```python
from build123d import *

# Parameters (mm, degrees)
SKETCH_1_R               = 25
SKETCH_1_R_2             = 12
EXTRUDE_1_DEPTH          = 10
SKETCH_2_R               = 25
SKETCH_2_R_2             = 4
EXTRUDE_2_DEPTH          = 10
SKETCH_5_W               = 37
SKETCH_5_H               = 20
EXTRUDE_3_DEPTH          = 25
CUT_EXTRUDE_1_DEPTH      = 20.184828
SKETCH_8_R               = 2
CUT_EXTRUDE_2_DEPTH      = 49.928519291
CUT_EXTRUDE_4_DEPTH      = 10
CUT_EXTRUDE_5_DEPTH      = 70.778220126
CUT_EXTRUDE_6_DEPTH      = 15.5
SKETCH_12_R              = 10
CUT_EXTRUDE_7_DEPTH      = 30
CUT_EXTRUDE_8_DEPTH      = 46.760244912
CUT_EXTRUDE_8_DEPTH_BACK = 46.760244912


with BuildPart() as part:
    # 草图1 → 凸台-拉伸1 (new body)
    with BuildSketch(Plane(origin=(0, 0, 0), x_dir=(1, 0, 0), z_dir=(0, 1, 0))):
        with Locations(Location((0, 0, 0), (0, 0, 270))):
            Circle(SKETCH_1_R)
        with Locations(Location((0, 0, 0), (0, 0, 270))):
            Circle(SKETCH_1_R_2, mode=Mode.SUBTRACT)
    extrude(amount=EXTRUDE_1_DEPTH)

    # 草图2 → 凸台-拉伸2 (add)
    with BuildSketch(Plane(origin=(0, 10, 0), x_dir=(1, 0, 0), z_dir=(0, 1, 0))):
        with Locations(Location((0, 0, 0), (0, 0, 270))):
            Circle(SKETCH_2_R)
        with Locations(Location((0, 0, 0), (0, 0, 270))):
            Circle(SKETCH_2_R_2, mode=Mode.SUBTRACT)
    extrude(amount=EXTRUDE_2_DEPTH)

    # 草图5 → 凸台-拉伸3 (add)
    with BuildSketch(Plane.XY.offset(12)):
        with Locations((0, 10)):
            Rectangle(SKETCH_5_W, SKETCH_5_H)
    extrude(amount=EXTRUDE_3_DEPTH)

    # 草图6 → 切除-拉伸1 (cut)
    with BuildSketch(Plane.XY.offset(37)):
        with BuildLine():
            Line((-18.490572983, -0.909482628), (-28.986413715, -0.909482628))
            Line((-28.986413715, -0.909482628), (-28.986413715, 31.85575571))
            Line((-28.986413715, 31.85575571), (34.685567791, 31.85575571))
            Line((34.685567791, 31.85575571), (34.685567791, -1.610938363))
            Line((34.685567791, -1.610938363), (18.499667367, -1.610938363))
            ThreePointArc((18.499667367, -1.610938363), (0.350757344, 16.996674547), (-18.490572983, -0.909482628))
        make_face()
    extrude(amount=-CUT_EXTRUDE_1_DEPTH, mode=Mode.SUBTRACT)

    # 草图8 → 切除-拉伸2 (cut, through all)
    with BuildSketch(Plane.XZ):
        with Locations(Location((18.75, 0, 0), (0, 0, 270))):
            Circle(SKETCH_8_R)
        with Locations(Location((13.258252147, 13.258252147, 0), (0, 0, 270))):
            Circle(SKETCH_8_R)
        with Locations(Location((0, 18.75, 0), (0, 0, 284.666911028))):
            Circle(SKETCH_8_R)
        with Locations(Location((-18.75, 0, 0), (0, 0, 90))):
            Circle(SKETCH_8_R)
        with Locations(Location((-13.258252147, 13.258252147, 0), (0, 0, 90))):
            Circle(SKETCH_8_R)
        with Locations(Location((13.258252147, -13.258252147, 0), (0, 0, 90))):
            Circle(SKETCH_8_R)
        with Locations(Location((0, -18.75, 0), (0, 0, 270))):
            Circle(SKETCH_8_R)
        with Locations(Location((-13.258252147, -13.258252147, 0), (0, 0, 270))):
            Circle(SKETCH_8_R)
    extrude(amount=-CUT_EXTRUDE_2_DEPTH, mode=Mode.SUBTRACT)

    # 草图9 → 切除-拉伸4 (cut)
    with BuildSketch(Plane(origin=(0, 0, 0), x_dir=(1, 0, 0), z_dir=(0, 1, 0))):
        Polygon((0, 0), (10.593685304, 25.575418736), (-10.593685304, 25.575418736), align=None)
    extrude(amount=CUT_EXTRUDE_4_DEPTH, mode=Mode.SUBTRACT)

    # 草图10 → 切除-拉伸5 (cut, through all)
    with BuildSketch(Plane.XY.offset(37)):
        with BuildLine():
            Line((-18.5, 6.099342077), (-25, 6.099342077))
            Line((-25, 6.099342077), (-25, 20))
            Line((-25, 20), (25, 20))
            Line((25, 20), (25, 6.099342077))
            Line((25, 6.099342077), (18.5, 6.099342077))
            ThreePointArc((18.5, 6.099342077), (0, 18.5), (-18.5, 6.099342077))
        make_face()
    extrude(amount=-CUT_EXTRUDE_5_DEPTH, mode=Mode.SUBTRACT)

    # 草图11 → 切除-拉伸6 (cut)
    with BuildSketch(Plane(origin=(0, 18.5, 0), x_dir=(1, 0, 0), z_dir=(0, 1, 0))):
        Polygon((0, -15.5), (-2.814582562, -17.125), (-2.814582562, -20.375), (0, -22), (2.814582562, -20.375), (2.814582562, -17.125), align=None)
        Polygon((-14.099414044, -10.118993212), (-10.960155108, -10.960155108), (-10.118993212, -14.099414044), (-12.417090251, -16.397511083), (-15.556349186, -15.556349186), (-16.397511083, -12.417090251), align=None)
        Polygon((10.960155108, -10.960155108), (10.118993212, -14.099414044), (12.417090251, -16.397511083), (15.556349186, -15.556349186), (16.397511083, -12.417090251), (14.099414044, -10.118993212), align=None)
        Polygon((-10.118993212, 14.099414044), (-10.960155108, 10.960155108), (-14.099414044, 10.118993212), (-16.397511083, 12.417090251), (-15.556349186, 15.556349186), (-12.417090251, 16.397511083), align=None)
        Polygon((-17.125, 2.814582562), (-15.5, 0), (-17.125, -2.814582562), (-20.375, -2.814582562), (-22, 0), (-20.375, 2.814582562), align=None)
        Polygon((10.960155108, 10.960155108), (14.099414044, 10.118993212), (16.397511083, 12.417090251), (15.556349186, 15.556349186), (12.417090251, 16.397511083), (10.118993212, 14.099414044), align=None)
        Polygon((15.5, 0), (17.125, -2.814582562), (20.375, -2.814582562), (22, 0), (20.375, 2.814582562), (17.125, 2.814582562), align=None)
        Polygon((2.814582562, 17.125), (0, 15.5), (-2.814582562, 17.125), (-2.814582562, 20.375), (0, 22), (2.814582562, 20.375), align=None)
    extrude(amount=-CUT_EXTRUDE_6_DEPTH, mode=Mode.SUBTRACT)

    # 草图12 → 切除-拉伸7 (cut)
    with BuildSketch(Plane.XY.offset(37)):
        Circle(SKETCH_12_R)
    extrude(amount=-CUT_EXTRUDE_7_DEPTH, mode=Mode.SUBTRACT)

    # 草图13 → 切除-拉伸8 (cut, two sides: drawn at the far end of the back side and taken through both)
    with BuildSketch(Plane.XZ.offset(-10).offset(-CUT_EXTRUDE_8_DEPTH_BACK)):
        with BuildLine():
            Line((0, 0), (-10, 7))
            ThreePointArc((-10, 7), (0, 12.206555616), (10, 7))
            Line((10, 7), (0, 0))
        make_face()
    extrude(amount=CUT_EXTRUDE_8_DEPTH + CUT_EXTRUDE_8_DEPTH_BACK, mode=Mode.SUBTRACT)


solid = part.part
```
Geometry: final body of the model. Coordinates: model frame, mm. A direction names the side the tool comes from. Round coordinates to 2 decimals unless told otherwise and drop trailing zeros. Write each loop counter-clockwise with the first axis right and the second up, starting at its lowest first coordinate (ties: lowest second). Pieces come first, ordered by that corner, then holes.
Item 1: Pin query (flat end, axial travel): P1, Ø1, axis at y = 12, z = 18.5, coming from the +X side; P2, Ø1.6, axis at x = 19, y = 4.5, coming from the -Z side; P3, Ø8, axis at x = 0.5, z = -2, coming from the -Y side. Return the tip coordinate at first contact, or that it passes through.
Item 2: Section query C-C (z = 33). Return loops of the section in (x, y).
Item 3: Section query A-A (y = 1.5). Return loops of the section in (x, z), plus the area to 3 significant figures.
Item 4: Material intervals for L1, parallel to Z at x = 0, y = 15.25; L2, parallel to Z at x = -11, y = 3.75; L3, parallel to X at y = 1.35, z = 0, sorted ascending.
Item 5: Section query B-B (x = -1). Return loops of the section in (y, z), plus the area to 3 significant figures.
Item 6: Set-up query: faces 3 (the face through (0.2, 10, 22.2)), 4 (the face through (-12.552, 9.2, 10.534)), 5 (the face through (7.045, 4.93, -17.008)). Return all of +Z, -Z, +X, -X, +Y, -Y with unobstructed straight access to the full face (end or side cutting, diameter ignored); none if empty.
Item 7: Mould query, pull axis X, two halves, no side actions, for faces 1 (the face through (-12, 13, 16.815)), 2 (the face through (16.301, 6.222, 1.388)). Classes: +X half, -X half, draft (parallel to the pull), parting line (faces both ways), or undercut.
Completed:
1. P1: stops at x = 13.16
1. P2: stops at z = -17.14
1. P3: stops at y = 10
2. outline: (-18.44, 0) - (-10, 0) arc R10 cw to (10, 0) - (18.44, 0) arc R18.5 ccw to start
3. outline: (-18.5, 16.82) arc R25 ccw to (-9.57, -23.1) - (-4.59, -11.09) arc R12 cw to (-9.83, 6.88) - (-10, 7) arc R12.21 cw to (-9.89, 7.16) - (-9.89, 37) - (-18.26, 37) - (-18.26, 16.82) - close; (4.59, -11.09) - (9.57, -23.1) arc R25 ccw to (18.5, 16.82) - (18.26, 16.82) - (18.26, 37) - (9.89, 37) - (9.89, 7.16) arc R12.21 cw to (10, 7) - (9.83, 6.88) arc R12 cw to start; hole circle Ø4 at (-18.75, 0); hole circle Ø4 at (-13.26, -13.26); hole circle Ø4 at (-13.26, 13.26); hole circle Ø4 at (13.26, -13.26); hole circle Ø4 at (13.26, 13.26); hole circle Ø4 at (18.75, 0)
3. area: 1,250 mm2
4. L1: z = -25 to -22, -15.5 to -4, 12.21 to 15.5, 22 to 37
4. L2: z = -22.45 to -14.98, -10.95 to -4.8, 4.8 to 10.95, 14.98 to 37
4. L3: x = -25 to -20.75, -16.75 to -12, 12 to 16.75, 20.75 to 25
5. outline: (9.95, 12.17) - (18.47, 12.17) - (18.47, 16.08) - (9.95, 16.08) - close; (9.95, 21.42) - (16.97, 21.42) - (16.97, 37) - (9.95, 37) - close; (10, -24.98) - (18.47, -24.98) - (18.47, -21.42) - (10, -21.42) - close; (10, -16.08) - (18.47, -16.08) - (18.47, -3.87) - (10, -3.87) - close
5. area: 276 mm2
6. face 3: +Z, -Y
6. face 4: +Y
6. face 5: -Z, -Y
7. face 1: draft
7. face 2: undercut
